The model under review builds one solid part; all positions refer to its coordinate system, in mm. Face numbers are marked on the shaded views. A direction names the side the tool comes from. Coordinates: 2 decimals unless noted, no trailing zeros. Order: outer loops, then holes, each group sorted by start corner. A loop starts at its lowest first (then second) coordinate and runs counter-clockwise, first axis right, second up.
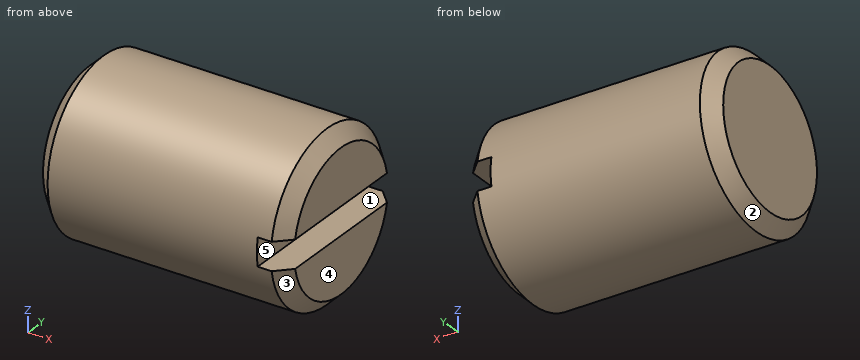
```python
from build123d import *

# Parameters (mm, degrees)
CROQUIS1_R              = 3
SALIENTE_EXTRUIR1_DEPTH = 9
CROQUIS2_W              = 1
CROQUIS2_H              = 7
CORTAR_EXTRUIR1_DEPTH   = 1
CHAFL_N1_SIZE           = 0.5


with BuildPart() as part:
    # Croquis1 → Saliente-Extruir1 (new body)
    with BuildSketch(Plane(origin=(0, 0, 0), x_dir=(0, 0, -1), z_dir=(1, 0, 0))):
        Circle(CROQUIS1_R)
    extrude(amount=SALIENTE_EXTRUIR1_DEPTH)

    # Croquis2 → Cortar-Extruir1 (cut)
    with BuildSketch(Plane(origin=(9, 0, 0), x_dir=(0, 0, -1), z_dir=(1, 0, 0))):
        Rectangle(CROQUIS2_W, CROQUIS2_H)
    extrude(amount=-CORTAR_EXTRUIR1_DEPTH, mode=Mode.SUBTRACT)

    # Chaflán1
    chafl_n1_edges = [part.edges().sort_by_distance(p)[0] for p in [
        (0, 0, 3),
        (9, 0, 3),
        (9, -1.936491673, -2.291287847),
    ]]
    chamfer(chafl_n1_edges, length=CHAFL_N1_SIZE)


solid = part.part
```
(1) We need section A-A, the plane y = 0. Write out the cut boundary in (x, z), and give its area (3 significant figures).
A:
outline: (0, -2.5) - (0.5, -3) - (8.5, -3) - (9, -2.5) - (9, -0.5) - (8, -0.5) - (8, 0.5) - (9, 0.5) - (9, 2.5) - (8.5, 3) - (0.5, 3) - (0, 2.5) - close
area: 52.5 mm2
(2) Draft analysis for pull direction Z (two halves, no side actions). For the marked faces 3, 4 and 5, state which applies: released by +Z, released by -Z, zero draft, split by the parting line, or undercut.
A:
face 3: released by -Z
face 4: zero draft
face 5: undercut
(3) We need section B-B, the plane z = 0. Write out the cut boundary in (x, y).
A:
outline: (0, -2.5) - (0.5, -3) - (8, -3) - (8, 3) - (0.5, 3) - (0, 2.5) - close
(4) For pin 1 Ø3 at (x, y) = (5, -0.5) entering from +Z; pin 2 Ø1 at (y, z) = (2.5, -2) entering from -X; pin 3 Ø1.5 at (x, z) = (5, 1) entering from -Y, all flat-tipped, find the tip position at first contact; note any pin that passes through.
A:
pin 1: stops at z = 3
pin 2: stops at x = 0.2
pin 3: stops at y = -2.99
(5) We need section C-C, the plane x = 1.75. Write out the cut boundary in (y, z), and give its area (3 significant figures).
A:
outline: circle Ø6 at (0, 0)
area: 28.3 mm2
(6) Machinability: for the marked faces 1 and 2, which of the approach directions +Z, -Z, +X, -X, +Y, -Y give a long, thin tool a straight path to every point of the face, cutting with its end or side? Answer none if there is none.
A:
face 1: +X, +Y, -Y
face 2: -X
(7) Wall thickness on probe 1 along Z at (x, y) = (1.5, 0.1); probe 2 along X at (y, z) = (-0.5, -0.1); probe 3 along Y at (x, z) = (3.25, 1): over which ranges is each line inside the solid? List them lowest first.
A:
probe 1: z = -3 to 3
probe 2: x = 0 to 8
probe 3: y = -2.83 to 2.83
